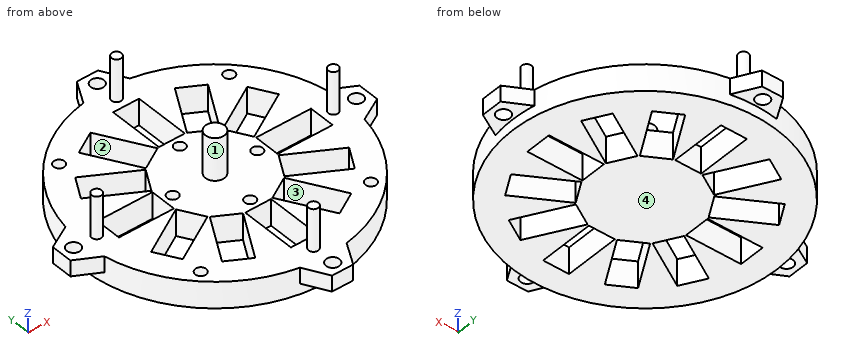
from build123d import *

# Parameters (mm, degrees)
CROQUIS2_R              = 50
SALIENTE_EXTRUIR1_DEPTH = 10
CROQUIS1_W              = 9.8
CROQUIS1_H              = 20.8
CROQUIS1_W_2            = 20.8
CROQUIS1_H_2            = 9.8
CORTAR_EXTRUIR3_DEPTH   = 72.414284285
CROQUIS4_R              = 3.6
SALIENTE_EXTRUIR2_DEPTH = 16
CROQUIS5_R              = 1.85
SALIENTE_EXTRUIR3_DEPTH = 16
SALIENTE_EXTRUIR4_START = -6
SALIENTE_EXTRUIR4_DEPTH = 6
CROQUIS8_R              = 2.5
CORTAR_EXTRUIR4_DEPTH   = 6.5
CROQUIS9_R              = 2.05
CORTAR_EXTRUIR5_DEPTH   = 6


with BuildPart() as part:
    # Croquis2 → Saliente-Extruir1 (new body)
    with BuildSketch(Plane(origin=(0, 0, 0), x_dir=(0, 1, 0), z_dir=(0, 0, 1))):
        with Locations(Location((0, 0, 0), (0, 0, 270))):
            Circle(CROQUIS2_R)
    extrude(amount=SALIENTE_EXTRUIR1_DEPTH)

    # Croquis1 → Cortar-Extruir3 (cut, through all)
    with BuildSketch(Plane(origin=(0, 0, 0), x_dir=(0, 1, 0), z_dir=(0, 0, 1))):
        Polygon((15.956475521, 37.437426313), (5.556475521, 19.424097914), (14.043524479, 14.524097914), (24.443524479, 32.537426313), align=None)
        with Locations((0, 30)):
            Rectangle(CROQUIS1_W, CROQUIS1_H)
        Polygon((32.537426313, 24.443524479), (14.524097914, 14.043524479), (19.424097914, 5.556475521), (37.437426313, 15.956475521), align=None)
        with Locations((30, 0)):
            Rectangle(CROQUIS1_W_2, CROQUIS1_H_2)
        Polygon((37.437426313, -15.956475521), (19.424097914, -5.556475521), (14.524097914, -14.043524479), (32.537426313, -24.443524479), align=None)
        Polygon((24.443524479, -32.537426313), (14.043524479, -14.524097914), (5.556475521, -19.424097914), (15.956475521, -37.437426313), align=None)
        with Locations((0, -30)):
            Rectangle(CROQUIS1_W, CROQUIS1_H)
        Polygon((-15.956475521, -37.437426313), (-5.556475521, -19.424097914), (-14.043524479, -14.524097914), (-24.443524479, -32.537426313), align=None)
        Polygon((-32.537426313, -24.443524479), (-14.524097914, -14.043524479), (-19.424097914, -5.556475521), (-37.437426313, -15.956475521), align=None)
        with Locations((-30, 0)):
            Rectangle(CROQUIS1_W_2, CROQUIS1_H_2)
        Polygon((-37.437426313, 15.956475521), (-19.424097914, 5.556475521), (-14.524097914, 14.043524479), (-32.537426313, 24.443524479), align=None)
        Polygon((-24.443524479, 32.537426313), (-14.043524479, 14.524097914), (-5.556475521, 19.424097914), (-15.956475521, 37.437426313), align=None)
    extrude(amount=CORTAR_EXTRUIR3_DEPTH, mode=Mode.SUBTRACT)

    # Croquis4 → Saliente-Extruir2 (add)
    with BuildSketch(Plane.XY.offset(10)):
        Circle(CROQUIS4_R)
    extrude(amount=SALIENTE_EXTRUIR2_DEPTH)

    # Croquis5 → Saliente-Extruir3 (add)
    with BuildSketch(Plane.XY.offset(10)):
        with Locations((0, 44.75)):
            Circle(CROQUIS5_R)
        with Locations((44.75, 0)):
            Circle(CROQUIS5_R)
        with Locations((0, -44.75)):
            Circle(CROQUIS5_R)
        with Locations((-44.75, 0)):
            Circle(CROQUIS5_R)
    extrude(amount=SALIENTE_EXTRUIR3_DEPTH)

    # Croquis7 → Saliente-Extruir4 (add)
    with BuildSketch(Plane.XY.offset(10).offset(SALIENTE_EXTRUIR4_START)):
        with BuildLine():
            Line((4, 58), (8.81247625, 49.217276056))
            ThreePointArc((8.81247625, 49.217276056), (0, 50), (-8.81247625, 49.217276056))
            Line((-8.81247625, 49.217276056), (-4, 58))
            Line((-4, 58), (4, 58))
        make_face()
        with BuildLine():
            Line((58, 4), (49.217276056, 8.81247625))
            ThreePointArc((49.217276056, 8.81247625), (50, 0), (49.217276056, -8.81247625))
            Line((49.217276056, -8.81247625), (58, -4))
            Line((58, -4), (58, 4))
        make_face()
        with BuildLine():
            Line((4, -58), (8.81247625, -49.217276056))
            ThreePointArc((8.81247625, -49.217276056), (0, -50), (-8.81247625, -49.217276056))
            Line((-8.81247625, -49.217276056), (-4, -58))
            Line((-4, -58), (4, -58))
        make_face()
        with BuildLine():
            Line((-58, -4), (-49.217276056, -8.81247625))
            ThreePointArc((-49.217276056, -8.81247625), (-50, 0), (-49.217276056, 8.81247625))
            Line((-49.217276056, 8.81247625), (-58, 4))
            Line((-58, 4), (-58, -4))
        make_face()
    extrude(amount=SALIENTE_EXTRUIR4_DEPTH)

    # Croquis8 → Cortar-Extruir4 (cut)
    with BuildSketch(Plane.XY.offset(10)):
        with Locations((0, 53.5)):
            Circle(CROQUIS8_R)
        with Locations((53.5, 0)):
            Circle(CROQUIS8_R)
        with Locations((0, -53.5)):
            Circle(CROQUIS8_R)
        with Locations((-53.5, 0)):
            Circle(CROQUIS8_R)
    extrude(amount=-CORTAR_EXTRUIR4_DEPTH, mode=Mode.SUBTRACT)

    # Croquis9 → Cortar-Extruir5 (cut)
    with BuildSketch(Plane.XY.offset(10)):
        with Locations((0, 16)):
            Circle(CROQUIS9_R)
        with Locations((16, 0)):
            Circle(CROQUIS9_R)
        with Locations((0, -16)):
            Circle(CROQUIS9_R)
        with Locations((-16, 0)):
            Circle(CROQUIS9_R)
        with Locations((-32.173358544, 32.173358544)):
            Circle(CROQUIS9_R)
        with Locations((32.173358544, 32.173358544)):
            Circle(CROQUIS9_R)
        with Locations((32.173358544, -32.173358544)):
            Circle(CROQUIS9_R)
        with Locations((-32.173358544, -32.173358544)):
            Circle(CROQUIS9_R)
    extrude(amount=-CORTAR_EXTRUIR5_DEPTH, mode=Mode.SUBTRACT)


solid = part.part
Geometry check sheet. Reference: the model listing, model coordinates, mm. Face numbers are marked on the shaded views. A direction names the side the tool comes from. Give positions to 0.01 mm unless a question says otherwise; leave off trailing zeros. Write each loop counter-clockwise with the first axis right and the second up, starting at its lowest first coordinate (ties: lowest second). Pieces come first, ordered by that corner, then holes. Notation, with made-up numbers: M -1.75,7 L 9.25,7 A19 ccw 9.25,11 Z; hole C -15.75,30.5 d3. An arc over 180 degrees is marked long. Answer as CSV lines item,"result". Start each with the question number.
Q1. Section check B-B, the plane z = 15. Record the cut outline in (x, y), then the cut area to 3 significant figures.
Q2. Release check for a two-part mould opening along Y. For the marked faces 3 and 4 record: pulls with the +Y half, pulls with the -Y half, needs draft (parallel to the pull), parting line crosses it, or undercut.
Q3. Go/stop test with flat-tipped pins: pin 1 (3.5 mm diameter, centred on x = -16, y = 0, fed in from +Z); pin 2 (3.5 mm diameter, centred on x = 15.5, y = 0, fed in from +Z); pin 3 (6 mm diameter, centred on x = -39.5, y = 37, fed in from +Z); pin 4 (7 mm diameter, centred on x = -4.5, y = 53.5, fed in from -Z). Record where each tip stops, or that it passes through.
Q4. Section check D-D, the plane x = -23. Record the cut outline in (y, z), then the cut area to 3 significant figures.
Q5. Material ranges on L1, parallel to X at y = 32, z = 9.25; L2, parallel to Y at x = 32.5, z = 4.25; L3, parallel to Y at x = 29, z = 9.75, recorded low to high.
Q6. Section check A-A, the plane x = -53.5. Record the cut outline in (y, z), then the cut area to 3 significant figures.
Q7. Tool access check on the marked faces 1 and 2. Record the directions out of +Z, -Z, +X, -X, +Y, -Y that give a thin tool (end or side, any length) a straight path to the whole face; none if there is none.
Geometry says:
1,outline,"C -44.75,0 d3.7; C 0,0 d7.2; C 0,-44.75 d3.7; C 0,44.75 d3.7; C 44.75,0 d3.7"
1,area,"83.7 mm^2"
2,face 3,"undercut"
2,face 4,"needs draft"
3,pin 1,"z = 4"
3,pin 2,"z = 10"
3,pin 3,"through"
3,pin 4,"z = 4"
4,outline,"M -44.4,0 L -33.37,0 L -33.37,10 L -44.4,10 Z; M -30.04,0 L -18.94,0 L -18.94,10 L -30.04,10 Z; M -7.62,0 L -4.9,0 L -4.9,10 L -7.62,10 Z; M 4.9,0 L 7.62,0 L 7.62,10 L 4.9,10 Z; M 18.94,0 L 30.04,0 L 30.04,10 L 18.94,10 Z; M 33.37,0 L 44.4,0 L 44.4,10 L 33.37,10 Z"
4,area,"497 mm^2"
5,L1,"-38.42 to -34.22, -30.13 to -24.13, -12.82 to -4.9, 4.9 to 12.82, 24.13 to 30.13, 34.22 to 38.42"
5,L2,"-38 to -34.2, -30.15 to -24.42, -13.11 to -4.9, 4.9 to 13.11, 24.42 to 30.15, 34.2 to 38"
5,L3,"-40.73 to -22.4, -11.09 to -4.9, 4.9 to 11.09, 22.4 to 40.73"
6,outline,"M -6.47,4 L -2.5,4 L -2.5,10 L -6.47,10 Z; M 2.5,4 L 6.47,4 L 6.47,10 L 2.5,10 Z"
6,area,"47.6 mm^2"
7,face 1,"+Z"
7,face 2,"+Z, -Z"
